For this review, use the dimensioned drawing (mm, ordinates from the lowest corner) and the shaded views. Give positions to 0.01 mm unless a question says otherwise; leave off trailing zeros. Loops run counter-clockwise (first coordinate to the right, second up) from the corner with the lowest first, then second, coordinate; pieces in that order, holes last. Notation, with made-up numbers: (-34.75, 79) -> (-8.75, 79) arc R9 cw to (-8.75, 96) -> close; hole circle Ø5 at (-24.75, 3.25). An arc over 180 degrees is marked (long way). Use a Markdown table: item, result. Add a question column.
1. For pin 1 Ø1 at (x, z) = (44.5, 1) entering from +Y; pin 2 Ø1 at (y, z) = (12, 1) entering from +X; pin 3 Ø5 at (x, y) = (25, 5) entering from -Z, all flat-tipped, find the tip position at first contact; note any pin that passes through.
2. Add section D-D (x = 8.5). State the section outline as (y, z) points, and give its area (3 significant figures).
3. To check wall thickness, follow line 1 (Y direction, x = 25, z = 0.95); line 2 (Y direction, x = 6, z = 0.4); line 3 (X direction, y = 11.75, z = 0.1). State the ranges of each line that lie inside material, in increasing order.
4. Add section C-C (y = 5). State the section outline as (x, z) points, and give its area (3 significant figures).
5. Add section B-B (z = 1.5). State the section outline as (x, y) points.
6. Add section A-A (x = 25). State the section outline as (y, z) points.
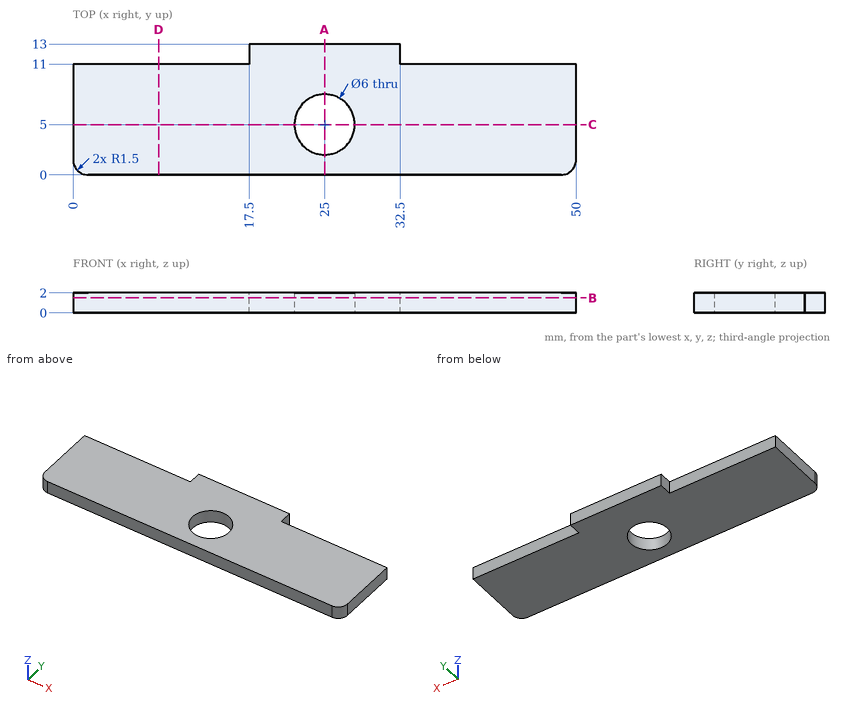
Taken from the geometry:
| question | item | result |
|---|---|---|
| 1 | pin 1 | stops at y = 11 |
| 1 | pin 2 | stops at x = 32.5 |
| 1 | pin 3 | passes through |
| 2 | outline | (0, 0) -> (11, 0) -> (11, 2) -> (0, 2) -> close |
| 2 | area | 22.0 mm^2 |
| 3 | line 1 | y = 0 to 2, 8 to 13 |
| 3 | line 2 | y = 0 to 11 |
| 3 | line 3 | x = 17.5 to 32.5 |
| 4 | outline | (0, 0) -> (22, 0) -> (22, 2) -> (0, 2) -> close; (28, 0) -> (50, 0) -> (50, 2) -> (28, 2) -> close |
| 4 | area | 88.0 mm^2 |
| 5 | outline | (0, 1.5) arc R1.5 ccw to (1.5, 0) -> (48.5, 0) arc R1.5 ccw to (50, 1.5) -> (50, 11) -> (32.5, 11) -> (32.5, 13) -> (17.5, 13) -> (17.5, 11) -> (0, 11) -> close; hole circle Ø6 at (25, 5) |
| 6 | outline | (0, 0) -> (2, 0) -> (2, 2) -> (0, 2) -> close; (8, 0) -> (13, 0) -> (13, 2) -> (8, 2) -> close |
